from build123d import *

# Parameters (mm, degrees)
F1_DEPTH = 25.4


with BuildPart() as f1:
    # F0 (on Right) → F1 (new body)
    with BuildSketch(Plane.YZ):
        with BuildLine():
            ThreePointArc((-91.4772798479, -11.9624281348), (-98.9167676057, 5.9980841073), (-116.8772798479, 13.4375718652))
            Line((-116.8772798479, 13.4375718652), (-116.8772798479, 0.7375718652))
            ThreePointArc((-116.8772798479, 0.7375718652), (-107.8970237268, -2.9821720138), (-104.1772798479, -11.9624281348))
            ThreePointArc((-104.1772798479, -11.9624281348), (-107.8970237268, -20.9426842559), (-116.8772798479, -24.6624281348))
            Line((-116.8772798479, -24.6624281348), (-116.8772798479, -37.3624281348))
            ThreePointArc((-116.8772798479, -37.3624281348), (-98.9167676057, -29.922940377), (-91.4772798479, -11.9624281348))
        make_face()
        with BuildLine():
            Line((391.1227201521, 13.4375718652), (-116.8772798479, 13.4375718652))
            ThreePointArc((-116.8772798479, 13.4375718652), (-98.9167676057, 5.9980841073), (-91.4772798479, -11.9624281348))
            ThreePointArc((-91.4772798479, -11.9624281348), (-98.9167676057, -29.922940377), (-116.8772798479, -37.3624281348))
            Line((-116.8772798479, -37.3624281348), (391.1227201521, -37.3624281348))
            ThreePointArc((391.1227201521, -37.3624281348), (365.7227201521, -11.9624281348), (391.1227201521, 13.4375718652))
        make_face()
        with BuildLine():
            Line((-116.8772798479, 0.7375718652), (-116.8772798479, 13.4375718652))
            ThreePointArc((-116.8772798479, 13.4375718652), (-142.2772798479, -11.9624281348), (-116.8772798479, -37.3624281348))
            Line((-116.8772798479, -37.3624281348), (-116.8772798479, -24.6624281348))
            ThreePointArc((-116.8772798479, -24.6624281348), (-129.5772798479, -11.9624281348), (-116.8772798479, 0.7375718652))
        make_face()
        with BuildLine():
            ThreePointArc((416.5227201521, -11.9624281348), (409.0832323943, 5.9980841073), (391.1227201521, 13.4375718652))
            Line((391.1227201521, 13.4375718652), (391.1227201521, 0.7375718652))
            ThreePointArc((391.1227201521, 0.7375718652), (400.1029762732, -2.9821720138), (403.8227201521, -11.9624281348))
            ThreePointArc((403.8227201521, -11.9624281348), (400.1029762732, -20.9426842559), (391.1227201521, -24.6624281348))
            Line((391.1227201521, -24.6624281348), (391.1227201521, -37.3624281348))
            ThreePointArc((391.1227201521, -37.3624281348), (409.0832323943, -29.922940377), (416.5227201521, -11.9624281348))
        make_face()
        with BuildLine():
            Line((391.1227201521, 0.7375718652), (391.1227201521, 13.4375718652))
            ThreePointArc((391.1227201521, 13.4375718652), (365.7227201521, -11.9624281348), (391.1227201521, -37.3624281348))
            Line((391.1227201521, -37.3624281348), (391.1227201521, -24.6624281348))
            ThreePointArc((391.1227201521, -24.6624281348), (378.4227201521, -11.9624281348), (391.1227201521, 0.7375718652))
        make_face()
    extrude(amount=F1_DEPTH)


solid = f1.part
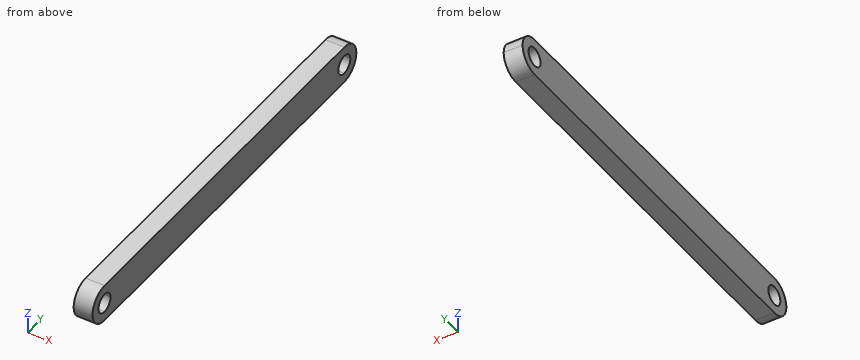
The model under review builds one solid part; all positions refer to its coordinate system, in mm. Round coordinates to 2 decimals unless told otherwise and drop trailing zeros. Loops run counter-clockwise (first coordinate to the right, second up) from the corner with the lowest first, then second, coordinate; pieces in that order, holes last. Notation, with made-up numbers: (16, 20) -> (53, 20) arc R16 cw to (53, 30) -> close; hole circle Ø5 at (9, -9.5). An arc over 180 degrees is marked (long way). One line per question, with ' | ' between items. Start each with the question number.
Item 1: Add section C-C, the plane z = 7.5. Write out the cut boundary in (x, y), then the cut area to 3 significant figures.
Item 2: Add section B-B, the plane z = -16.5. Write out the cut boundary in (x, y).
Item 3: For pin 1 (1.5 mm diameter, centred on x = 16, z = -12, fed in from -Y), flat-tipped, find the tip position at first contact; note if it passes through.
Item 4: Wall thickness on line 1 along Y through (x, z) = (13.5, -14.5); line 2 along Y through (x, z) = (1.75, -29.5); line 3 along Y through (x, z) = (22.25, 4.5): over which ranges is each line inside the solid? List them lowest first. Write a range as [from, to].
Item 5: Add section A-A, the plane x = 10.25. Write out the cut boundary in (y, z).
Return value:
1) outline: (0, -133.2) -> (25.4, -133.2) -> (25.4, 407.44) -> (0, 407.44) -> close | area: 13,700 mm2
2) outline: (0, -141.87) -> (25.4, -141.87) -> (25.4, -128.74) -> (0, -128.74) -> close; (0, -105.02) -> (25.4, -105.02) -> (25.4, 379.26) -> (0, 379.26) -> close; (0, 402.98) -> (25.4, 402.98) -> (25.4, 416.11) -> (0, 416.11) -> close
3) pin 1: stops at y = -142.28
4) line 1: y = [-142.15, -129.32], [-104.43, 378.68], [403.57, 416.4] | line 2: y = [-135.25, 409.5] | line 3: y = [-136.22, 410.47]
5) outline: (-116.88, -37.36) -> (391.12, -37.36) arc R25.4 ccw to (391.12, 13.44) -> (-116.88, 13.44) arc R25.4 ccw to start; hole circle Ø25.4 at (-116.88, -11.96); hole circle Ø25.4 at (391.12, -11.96)
